CAD build for the part. Positions are in the model's coordinates, mm. Face numbers are marked on the shaded views. Round coordinates to 2 decimals unless told otherwise and drop trailing zeros. Loops run counter-clockwise (first coordinate to the right, second up) from the corner with the lowest first, then second, coordinate; pieces in that order, holes last. Notation, with made-up numbers: M -32,81.25 L -20,81.25 A37 ccw -20,120.25 Z; hole C -28.75,22.5 d1. An arc over 180 degrees is marked long. Use a Markdown table: item, result. Add a question column.
(1) Wall check: L1, parallel to X at y = 95, z = 9.5; L2, parallel to X at y = 86, z = 9; L3, parallel to X at y = 157, z = 11. Give the ranges that are in metal, low to high.
(2) Flat gauge pins, fed straight in: P1, Ø1.5, axis at y = 156.5, z = 10.5, coming from the -X side; P2, Ø1, axis at y = 158, z = 5, coming from the -X side; P3, Ø5, axis at x = 85, z = 5, coming from the +Y side. Where does each tip first touch, or does it go through?
(3) Band-saw the part on A-A, the plane z = 7. Give the number of separate pieces and of enclosed holes in the cut face, and give its area (3 significant figures).
(4) Band-saw the part on B-B, the plane y = 102. Write the cut outline in (x, z), and give its area (3 significant figures).
(5) Two-plate mould, pull along Y, no slides. Class the marked faces 1 and 2: released by +Y, released by -Y, zero draft, split by the parting line, or undercut.
(6) Band-saw the part on C-C, the plane x = -54. Write the cut outline in (y, z).
(7) Band-saw the part on D-D, the plane y = 127. Write the cut outline in (x, z).
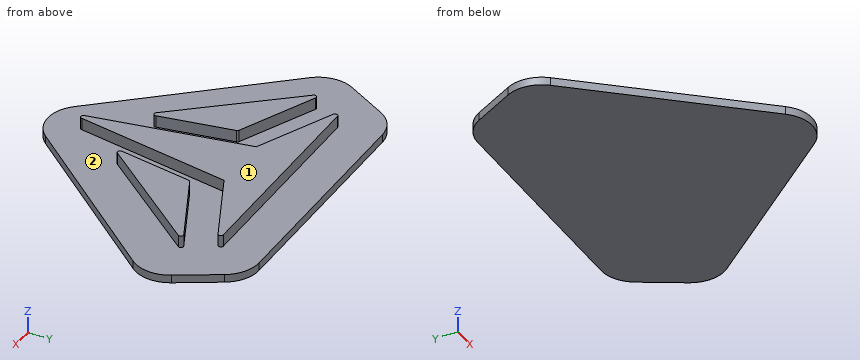
Autodesk Inventor part; units mm, degrees
ref_plane "YZ Plane" through (0, 0, 0) normal (1, 0, 0) x (0, 1, 0)
ref_plane "XZ Plane" through (0, 0, 0) normal (0, 1, 0) x (-1, 0, 0)
ref_plane "XY Plane" through (0, 0, 0) normal (0, 0, 1) x (1, 0, 0)
sketch "Sketch1" plane through (0, 0, 0) normal (0, 0, 1) x (1, 0, 0)
  line L0 (0, 184.15) -> (0, 133.3527) construction
  line L1 (0, 133.3527) -> (114.3119, 133.3527) construction
  line L2 (0, 133.3527) -> (-114.2939, 133.3527) construction
  line L3 (0, 184.15) -> (85.7282, 184.15)
  line L4 (0, 184.15) -> (-85.7274, 184.15)
  line L5 (-85.7274, 184.15) -> (-114.2939, 133.3527)
  line L6 (0, 0) -> (-114.2939, 133.3527)
  line L7 (0, 0) -> (114.3119, 133.3527)
  line L8 (85.7282, 184.15) -> (114.3119, 133.3527)
  line L9 (0, 158.7514) -> (0, 25.4014) construction
  line L10 (0, 158.7514) -> (74.6202, 158.7514)
  line L11 (0, 158.7514) -> (-74.6202, 158.7514)
  line L12 (0, 133.3527) -> (19.05, 133.3527) construction
  line L13 (0, 133.3527) -> (-19.05, 133.3527) construction
  line L14 (74.6202, 158.7514) -> (19.05, 133.3527)
  line L15 (19.05, 133.3527) -> (0, 25.4014)
  line L16 (0, 25.4014) -> (-19.05, 133.3527)
  line L17 (-74.6202, 158.7514) -> (-19.05, 133.3527)
  dimension "d0" = 184.15
  dimension "d1" = 19.05
  dimension "d2" = 19.05
sketch "Sketch2" plane through (0, 0, 0) normal (0, 0, 1) x (1, 0, 0)
  line L0 (74.6202, 158.7513) -> (83.9607, 142.1546) construction
  line L1 (19.05, 133.3527) -> (28.3932, 116.7512) construction
  line L2 (0, 0) -> (0, 63.5079) construction
  line L3 (0, 63.5079) -> (19.05, 63.5079) construction
  line L4 (19.05, 63.5079) -> (28.3932, 116.7512)
  line L5 (83.9607, 142.1546) -> (28.3932, 116.7512)
  line L6 (83.9607, 142.1546) -> (19.05, 63.5079)
  line L7 (-19.05, 63.5079) -> (-28.3932, 116.7512)
  line L8 (-83.9607, 142.1546) -> (-28.3932, 116.7512)
  line L9 (-83.9607, 142.1546) -> (-19.05, 63.5079)
  line L10 (74.6202, 158.7513) -> (0, 158.7513)
  line L11 (19.05, 133.3527) -> (74.6202, 158.7513)
  line L12 (0, 25.4018) -> (19.05, 133.3527)
  line L13 (0, 158.7513) -> (0, 25.4018) construction
  line L14 (-74.6202, 158.7513) -> (0, 158.7513)
  line L15 (-19.05, 133.3527) -> (-74.6202, 158.7513)
  line L16 (0, 25.4018) -> (-19.05, 133.3527)
  dimension "d3" = 19.05
extrude "Extrusion1" add sketch "Sketch1" along normal blind 5.08 contours L3 L8 L7 L6 L5 L4 | L10 L14 L15 L16 L17 L11
extrude "Extrusion2" add sketch "Sketch2" along normal blind 12.7
fillet "Fillet1" radius 22.225 5 edges at (114.3119, 133.3527, 2.54) (85.7282, 184.15, 2.54) (-85.7274, 184.15, 2.54) (-114.2939, 133.3527, 2.54) (0, 0, 2.54)
fillet "Fillet2" radius 1.5875 1 edges at (74.6202, 158.7513, 8.89)
fillet "Fillet3" radius 1.5875 1 edges at (0, 25.4018, 8.89)
fillet "Fillet4" radius 1.5875 1 edges at (-74.6202, 158.7513, 8.89)
fillet "Fillet5" radius 1.5875 4 edges at (-83.9607, 142.1546, 8.89) (83.9607, 142.1546, 8.89) (-19.05, 63.5079, 8.89) (19.05, 63.5079, 8.89)
fillet "Fillet6" radius 1.5875 2 edges at (28.3932, 116.7512, 8.89) (-28.3932, 116.7512, 8.89)
sketch "Sketch3" plane through (0, 0, 5.08) normal (0, 0, 1) x (1, 0, 0)
  point P0 (0, 0)
properties part number "item"
Return value:
| question | item | result |
|---|---|---|
| 1 | L1 | -45.04 to -24.58, -12.28 to 12.28, 24.58 to 45.04 |
| 1 | L2 | -37.61 to -23, -10.69 to 10.69, 23 to 37.61 |
| 1 | L3 | -68.91 to 68.91 |
| 2 | P1 | x = -68.92 |
| 2 | P2 | x = -100.71 |
| 2 | P3 | y = 181.89 |
| 3 | separate pieces | 3 |
| 3 | enclosed holes | 0 |
| 3 | area | 7,100 mm^2 |
| 4 | outline | M -87.42,0 L 87.44,0 L 87.44,5.08 L 50.82,5.08 L 50.82,12.7 L 25.8,12.7 L 25.8,5.08 L 13.52,5.08 L 13.52,12.7 L -13.52,12.7 L -13.52,5.08 L -25.8,5.08 L -25.8,12.7 L -50.82,12.7 L -50.82,5.08 L -87.42,5.08 Z |
| 4 | area | 1,480 mm^2 |
| 5 | face 1 | zero draft |
| 5 | face 2 | undercut |
| 6 | outline | M 63,0 L 184.15,0 L 184.15,5.08 L 158.75,5.08 L 158.75,12.7 L 149.33,12.7 L 149.33,5.08 L 128.46,5.08 L 128.46,12.7 L 105.85,12.7 L 105.85,5.08 L 63,5.08 Z |
| 7 | outline | M -107.62,0 L 107.63,0 L 107.63,5.08 L 71.45,5.08 L 71.45,12.7 L 50.81,12.7 L 50.81,5.08 L 17.93,5.08 L 17.93,12.7 L -17.93,12.7 L -17.93,5.08 L -50.81,5.08 L -50.81,12.7 L -71.45,12.7 L -71.45,5.08 L -107.62,5.08 Z |
